```python
from build123d import *

# Parameters (mm, degrees)
F0_W     = 8.1
F0_H     = 3.25
F0_R     = 1.5
F0_R_2   = 4
F0_R_3   = 18
F1_DEPTH = 3


with BuildPart() as f1:
    # F0 (on Front) → F1 (new body)
    with BuildSketch(Plane.XZ):
        Polygon((-62.5, -20.833333), (-62.5, -62.5), (-20.833333, -62.5), (-20.833333, -59.5), (20.833333, -59.5), (20.833333, -62.5), (62.5, -62.5), (62.5, -20.833333), (59.5, -20.833333), (59.5, 20.833333), (62.5, 20.833333), (62.5, 62.5), (20.833333, 62.5), (20.833333, 59.5), (-20.833333, 59.5), (-20.833333, 62.5), (-62.5, 62.5), (-62.5, 20.833333), (-59.5, 20.833333), (-59.5, -20.833333), align=None)
        with Locations((-24.05, -8.125)):
            Rectangle(F0_W, F0_H, mode=Mode.SUBTRACT)
        with Locations((0, -52.2)):
            Circle(F0_R, mode=Mode.SUBTRACT)
        with Locations((0, -35)):
            Circle(F0_R_2, mode=Mode.SUBTRACT)
        with Locations((24.05, -8.125)):
            Rectangle(F0_W, F0_H, mode=Mode.SUBTRACT)
        with Locations((-52.2, 0)):
            Circle(F0_R, mode=Mode.SUBTRACT)
        Circle(F0_R_3, mode=Mode.SUBTRACT)
        with Locations((52.2, 0)):
            Circle(F0_R, mode=Mode.SUBTRACT)
        with Locations((0, 52.2)):
            Circle(F0_R, mode=Mode.SUBTRACT)
    extrude(amount=F1_DEPTH)


with BuildPart() as f2_1:
    # F2: copy of F1
    add(f1.part.moved(Location((0, 60, 0))))


solid = f1.part
```
CAD build for the part. Positions are in the model's coordinates, mm. A direction names the side the tool comes from. Coordinates: 2 decimals unless noted, no trailing zeros. Order: outer loops, then holes, each group sorted by start corner. A loop starts at its lowest first (then second) coordinate and runs counter-clockwise, first axis right, second up. Notation, with made-up numbers: (37.5, 7) - (80.5, 7) arc R18 ccw to (80.5, 24) - close; hole circle Ø3 at (-36, -16.75). An arc over 180 degrees is marked (long way). Answer in a Markdown table with one row per item.
1. 3-axis set-ups, long thin cutter, end or side, ignore diameter. For faces 1 (the face through (-61, -1, 20.833)), 2 (the face through (24, -1, -9.75)), 3 (the face through (59.5, -1, 0)), 4 (the face through (-20.833, -1, 61)), 5 (the face through (0, -1, -59.5)): which of +Z, -Z, +X, -X, +Y, -Y reach the whole face in a straight line?
Answer:
| item | result |
|---|---|
| face 1 | -X, +Y, -Y |
| face 2 | +Y, -Y |
| face 3 | +X, +Y, -Y |
| face 4 | +Z, +Y, -Y |
| face 5 | -Z, +Y, -Y |
2. Slice it at C-C, the plane x = 0. List the corners of the cut face in (y, z).
Answer:
| item | result |
|---|---|
| outline | (-3, -59.5) - (0, -59.5) - (0, -53.7) - (-3, -53.7) - close; (-3, -50.7) - (0, -50.7) - (0, -39) - (-3, -39) - close; (-3, -31) - (0, -31) - (0, -18) - (-3, -18) - close; (-3, 18) - (0, 18) - (0, 50.7) - (-3, 50.7) - close; (-3, 53.7) - (0, 53.7) - (0, 59.5) - (-3, 59.5) - close |
3. Flat gauge pins, fed straight in: P1, Ø4, axis at x = 14.5, z = 3.5, coming from the +Y side; P2, Ø1.5, axis at x = -1, y = -2, coming from the -Z side; P3, Ø1.5, axis at y = -2, z = -8.5, coming from the +X side. Where does each tip first touch, or does it go through?
Answer:
| item | result |
|---|---|
| P1 | through |
| P2 | z = -59.5 |
| P3 | x = 59.5 |
4. Slice it at A-A, the plane x = -52.2. List the corners of the cut face in (y, z), then the cut area to 3 significant figures.
Answer:
| item | result |
|---|---|
| outline | (-3, -62.5) - (0, -62.5) - (0, -1.5) - (-3, -1.5) - close; (-3, 1.5) - (0, 1.5) - (0, 62.5) - (-3, 62.5) - close |
| area | 366 mm² |
5. Drill centre lines: L1, parallel to Z at x = 0, y = -1.75; L2, parallel to Z at x = -52.2, y = -1; L3, parallel to X at y = -2.7, z = -0.5. Where is each one in solid material? Low to high. Write a range as from..to.
Answer:
| item | result |
|---|---|
| L1 | -59.5..-53.7, -50.7..-39, -31..-18, 18..50.7, 53.7..59.5 |
| L2 | -62.5..-1.5, 1.5..62.5 |
| L3 | -59.5..-53.61, -50.79..-17.99, 17.99..50.79, 53.61..59.5 |
6. Slice it at B-B, the plane z = -35. List the corners of the cut face in (x, y), then the cut area to 3 significant figures.
Answer:
| item | result |
|---|---|
| outline | (-62.5, -3) - (-4, -3) - (-4, 0) - (-62.5, 0) - close; (4, -3) - (62.5, -3) - (62.5, 0) - (4, 0) - close |
| area | 351 mm² |
7. Slice it at D-D, the plane y = -0.65. Give the number of separate pieces and of enclosed holes in the cut face, then the cut area to 3 significant figures.
Answer:
| item | result |
|---|---|
| separate pieces | 1 |
| enclosed holes | 8 |
| area | 14,000 mm² |
